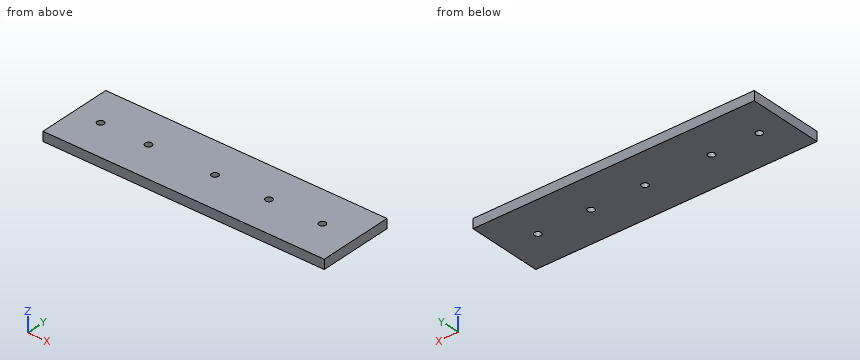
from build123d import *

# Parameters (mm, degrees)
F0_W     = 150
F0_H     = 40
F1_DEPTH = 2.5
F2_R     = 1.8
F3_DEPTH = 8


with BuildPart() as f1:
    # F0 (on Top) → F1 (new body, symmetric)
    with BuildSketch(Plane.XY):
        Rectangle(F0_W, F0_H)
    extrude(amount=F1_DEPTH, both=True)

    # F2 (on face) → F3 (cut)
    with BuildSketch(Plane.XY.offset(2.5)):
        with Locations((57.234262, 0)):
            Circle(F2_R)
        with Locations((28.762519, 0)):
            Circle(F2_R)
        Circle(F2_R)
        with Locations((-35.476741, 0)):
            Circle(F2_R)
        with Locations((-60.998922, 0)):
            Circle(F2_R)
    extrude(amount=-F3_DEPTH, mode=Mode.SUBTRACT)


solid = f1.part
Verification items for the finished model (mm, model axes). Give positions to 0.01 mm unless a question says otherwise; leave off trailing zeros. Write each loop counter-clockwise with the first axis right and the second up, starting at its lowest first coordinate (ties: lowest second). Pieces come first, ordered by that corner, then holes. Notation, with made-up numbers: (-37, 34.5) -> (-1, 34.5) arc R25 cw to (-1, 59.5) -> close; hole circle Ø4 at (40.25, -11). An arc over 180 degrees is marked (long way). Use CSV: the item, a comma, the result in double quotes.
(1) Sectioned sample at A-A (x = 0). Record the cut outline in (y, z), plus the area to 3 significant figures.
Derived:
outline,"(-20, -2.5) -> (-1.8, -2.5) -> (-1.8, 2.5) -> (-20, 2.5) -> close; (1.8, -2.5) -> (20, -2.5) -> (20, 2.5) -> (1.8, 2.5) -> close"
area,"182 mm^2"
(2) Sectioned sample at B-B (y = 0). Record the cut outline in (x, z).
Derived:
outline,"(-75, -2.5) -> (-62.8, -2.5) -> (-62.8, 2.5) -> (-75, 2.5) -> close; (-59.2, -2.5) -> (-37.28, -2.5) -> (-37.28, 2.5) -> (-59.2, 2.5) -> close; (-33.68, -2.5) -> (-1.8, -2.5) -> (-1.8, 2.5) -> (-33.68, 2.5) -> close; (1.8, -2.5) -> (26.96, -2.5) -> (26.96, 2.5) -> (1.8, 2.5) -> close; (30.56, -2.5) -> (55.43, -2.5) -> (55.43, 2.5) -> (30.56, 2.5) -> close; (59.03, -2.5) -> (75, -2.5) -> (75, 2.5) -> (59.03, 2.5) -> close"
(3) Sectioned sample at C-C (x = 57). Record the cut outline in (y, z), plus the area to 3 significant figures.
Derived:
outline,"(-20, -2.5) -> (-1.78, -2.5) -> (-1.78, 2.5) -> (-20, 2.5) -> close; (1.78, -2.5) -> (20, -2.5) -> (20, 2.5) -> (1.78, 2.5) -> close"
area,"182 mm^2"
(4) Go/stop test with flat-tipped pins: pin 1 (3 mm diameter, centred on x = -35.48, y = 0, fed in from +Z); pin 2 (4 mm diameter, centred on x = 57.23, y = 0, fed in from -Z). Record where each tip stops, or that it passes through.
Derived:
pin 1,"passes through"
pin 2,"stops at z = -2.5"
(5) Material ranges on L1, parallel to X at y = 0.5, z = -1.3; L2, parallel to X at y = 1, z = -0.95; L3, parallel to Y at x = 0, z = -0.95, recorded low to high.
Derived:
L1,"x = -75 to -62.73, -59.27 to -37.21, -33.75 to -1.73, 1.73 to 27.03, 30.49 to 55.51, 58.96 to 75"
L2,"x = -75 to -62.5, -59.5 to -36.97, -33.98 to -1.5, 1.5 to 27.27, 30.26 to 55.74, 58.73 to 75"
L3,"y = -20 to -1.8, 1.8 to 20"
